from build123d import *

# Parameters (mm, degrees)
BOSS_EXTRUDE1_DEPTH = 5.2832
CHAMFER1_SIZE       = 3.81


with BuildPart() as part:
    # Sketch1 → Boss-Extrude1 (new body)
    with BuildSketch(Plane.XY):
        Polygon((0, 0), (203.2, 0), (157.48, 68.834), (76.2, 68.834), align=None)
    extrude(amount=BOSS_EXTRUDE1_DEPTH)

    # Chamfer1
    # the kernel refuses this chamfer: 3.81 mm, written as the material it takes off along each edge
    with BuildSketch(Plane(origin=(208.621106578, -8.161777125, 5.2832), x_dir=(0.022903923995424024, 0.015212938447145094, -0.9996219169112966), z_dir=(-0.5532807214186398, 0.8329948639136195, 0))) as chamfer1_piece_1:
        Polygon((CHAMFER1_SIZE * 0.999621916911, CHAMFER1_SIZE * 0.0274958766106), (-CHAMFER1_SIZE * 0.0274958766106, CHAMFER1_SIZE * 0.999621916911), (0, 0), align=None)
    extrude(amount=102.230587414, mode=Mode.SUBTRACT)
    with BuildSketch(Plane(origin=(208.621106578, -8.161777125, 0), x_dir=(0.022903923995424024, 0.015212938447145094, 0.9996219169112966), z_dir=(-0.5532807214186398, 0.8329948639136195, 0))) as chamfer1_piece_2:
        Polygon((CHAMFER1_SIZE * 0.999621916911, -CHAMFER1_SIZE * 0.0274958766106), (-CHAMFER1_SIZE * 0.0274958766106, -CHAMFER1_SIZE * 0.999621916911), (0, 0), align=None)
    extrude(amount=102.230587414, mode=Mode.SUBTRACT)
    with BuildSketch(Plane(origin=(83.470816045, 75.401970494, 5.2832), x_dir=(-0.01843131645089907, 0.020403671347858754, -0.9996219169112968), z_dir=(-0.7420629513591385, -0.6703301993944216, 0))) as chamfer1_piece_3:
        Polygon((CHAMFER1_SIZE * 0.999621916911, CHAMFER1_SIZE * 0.0274958766106), (-CHAMFER1_SIZE * 0.0274958766106, CHAMFER1_SIZE * 0.999621916911), (0, 0), align=None)
    extrude(amount=122.282930207, mode=Mode.SUBTRACT)
    with BuildSketch(Plane(origin=(83.470816045, 75.401970494, 0), x_dir=(-0.01843131645089907, 0.020403671347858754, 0.9996219169112968), z_dir=(-0.7420629513591385, -0.6703301993944216, 0))) as chamfer1_piece_4:
        Polygon((CHAMFER1_SIZE * 0.999621916911, -CHAMFER1_SIZE * 0.0274958766106), (-CHAMFER1_SIZE * 0.0274958766106, -CHAMFER1_SIZE * 0.999621916911), (0, 0), align=None)
    extrude(amount=122.282930207, mode=Mode.SUBTRACT)


solid = part.part
Can you work these out from the model? Positions are in its coordinate system, mm. Coordinates: 2 decimals unless noted, no trailing zeros. Write each loop counter-clockwise with the first axis right and the second up, starting at its lowest first coordinate (ties: lowest second). Pieces come first, ordered by that corner, then holes. Notation, with made-up numbers: (34.25, 77.25) - (78.25, 77.25) arc R17 cw to (78.25, 84.25) - close; hole circle Ø6 at (-23.5, -12). An arc over 180 degrees is marked (long way). Return JSON: item names as keys, results as strings. Group by question number.
Item 1: If we section it at B-B (y = 20.5): Write out the boundary of the cut face in (x, z), then the cut area to 3 significant figures.
Item 2: If we section it at D-D (y = 11.5): Write out the boundary of the cut face in (x, z), then the cut area to 3 significant figures.
Item 3: Please list where these lines run through material, in increasing order: probe 1 along X at (y, z) = (44, 1.45); probe 2 along Y at (x, z) = (50, 3.9); probe 3 along X at (y, z) = (19, 3.85).
Item 4: I'm going to push a flat-ended pin straight in: pin 1 Ø2 at (y, z) = (35.5, 1) entering from -X. Where does the tip first touch, or does it pass through?
Item 5: If we section it at A-A (x = 175.5): Write out the boundary of the cut face in (y, z), then the cut area to 3 significant figures.
Item 6: If we section it at C-C (z = 1.75): Write out the boundary of the cut face in (x, y).
Return value:
{
 "1": {"outline": "(24.44, 2.64) - (28.38, 0) - (185.01, 0) - (188.18, 2.64) - (185.01, 5.28) - (28.38, 5.28) - close", "area": "846 mm^2"},
 "2": {"outline": "(14.47, 2.64) - (18.41, 0) - (190.99, 0) - (194.16, 2.64) - (190.99, 5.28) - (18.41, 5.28) - close", "area": "931 mm^2"},
 "3": {"probe 1": "x = 52.23 to 171.14", "probe 2": "y = 0 to 41.9", "probe 3": "x = 24.58 to 187.73"},
 "4": {"pin 1": "stops at x = 41.63"},
 "5": {"outline": "(0, 0) - (34.82, 0) - (39.59, 2.64) - (34.82, 5.28) - (0, 5.28) - close", "area": "197 mm^2"},
 "6": {"outline": "(3.07, 0) - (200.73, 0) - (155.01, 68.83) - (79.27, 68.83) - close"}
}
